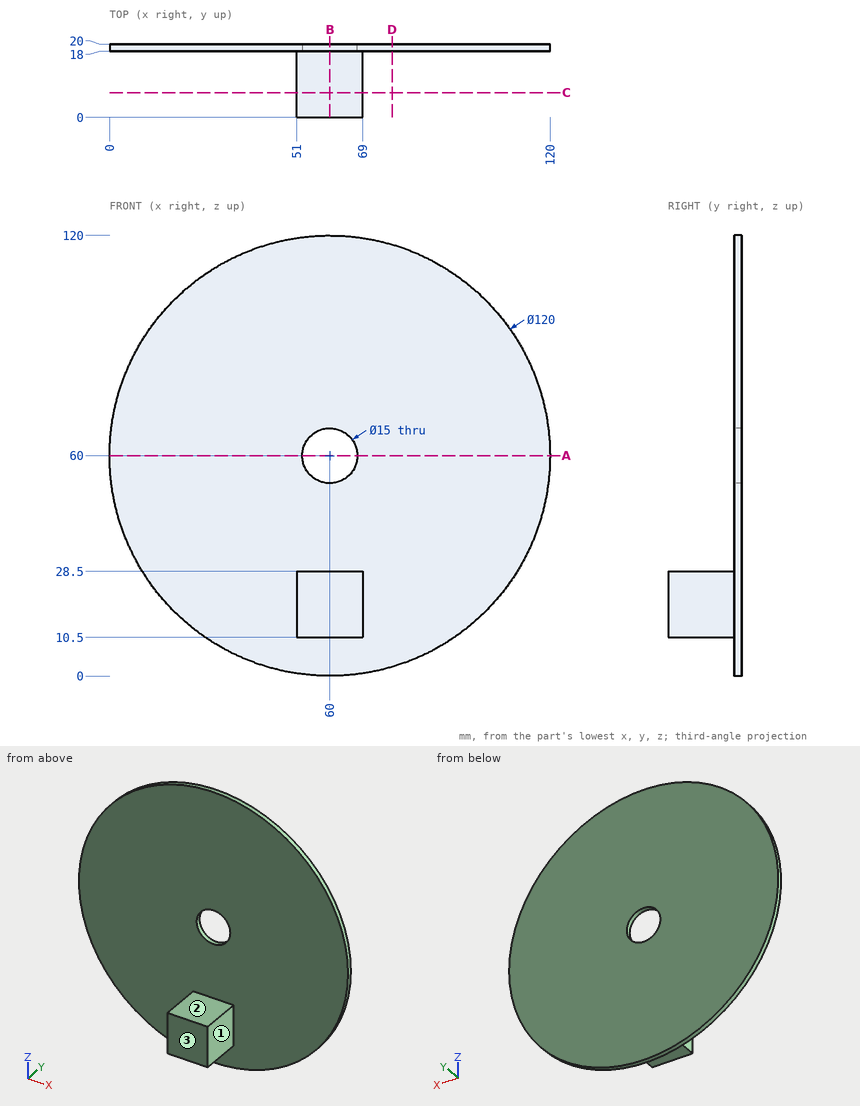
Job drawing, mm, ordinate dimensions from the low corner. One solid piece. A direction names the side the tool comes from. Coordinates: 2 decimals unless noted, no trailing zeros. Order: outer loops, then holes, each group sorted by start corner. A loop starts at its lowest first (then second) coordinate and runs counter-clockwise, first axis right, second up. Notation, with made-up numbers: (65, 26.25) - (97, 26.25) arc R27 cw to (97, 43.25) - close; hole circle Ø11 at (65.5, -13.75). An arc over 180 degrees is marked (long way). Return JSON: item names as keys, results as strings. Group by question number.
1) Saw through at D-D, the plane x = 77. Write the cut outline in (y, z).
2) Probe line 1 (X direction, y = 18.65, z = 60); line 2 (Y direction, x = 86, z = 112.5). List the from-to ranges inside material, lowest first. Write a range as from..to.
3) Saw through at A-A, the plane z = 60. Write the cut outline in (x, y), plus the area to 3 significant figures.
4) Saw through at B-B, the plane x = 60. Write the cut outline in (y, z).
5) Saw through at C-C, the plane y = 6.75. Write the cut outline in (x, z).
6) Tool access for the marked faces 1, 2 and 3: list every direction of +Z, -Z, +X, -X, +Y, -Y with a clear straight run to the whole face (end or side of a thin tool).
7) Flat gauge pins, fed straight in: P1, Ø12, axis at x = 28, z = 104, coming from the -Y side; P2, Ø4, axis at x = 58.5, y = 15.5, coming from the -Z side; P3, Ø10, axis at x = 54.5, y = 14, coming from the +Z side. Where does each tip first touch, or does it go through?
Values found:
{
 "1": {"outline": "(18, 2.46) - (20, 2.46) - (20, 117.54) - (18, 117.54) - close"},
 "2": {"line 1": "x = 0..52.5, 67.5..120", "line 2": "y = 18..20"},
 "3": {"outline": "(0, 18) - (52.5, 18) - (52.5, 20) - (0, 20) - close; (67.5, 18) - (120, 18) - (120, 20) - (67.5, 20) - close", "area": "210 mm²"},
 "4": {"outline": "(0, 10.5) - (18, 10.5) - (18, 0) - (20, 0) - (20, 52.5) - (18, 52.5) - (18, 28.5) - (0, 28.5) - close; (18, 67.5) - (20, 67.5) - (20, 120) - (18, 120) - close"},
 "5": {"outline": "(51, 10.5) - (69, 10.5) - (69, 28.5) - (51, 28.5) - close"},
 "6": {"face 1": "+Z, -Z, +X, -Y", "face 2": "+Z, +X, -X, -Y", "face 3": "+Z, -Z, +X, -X, -Y"},
 "7": {"P1": "stops at y = 18", "P2": "stops at z = 10.5", "P3": "stops at z = 119.95"}
}
